Geometry: final body of the model. Coordinates: model frame, mm. A direction names the side the tool comes from. Coordinates: 2 decimals unless noted, no trailing zeros. Order: outer loops, then holes, each group sorted by start corner. A loop starts at its lowest first (then second) coordinate and runs counter-clockwise, first axis right, second up. Notation, with made-up numbers: (59.25, 81.25) -> (100.25, 81.25) arc R8 ccw to (100.25, 88.25) -> close; hole circle Ø6 at (-28, 12.5). An arc over 180 degrees is marked (long way). Answer in a Markdown table with one row per item. Add a question column.
1) Contact query for flat-ended pins moving along their axis: P1, Ø3, axis at x = 4.5, z = 1279, coming from the +Y side; P2, Ø3, axis at x = -44, y = 633.5, coming from the -Z side (3 decimals); P3, Ø6.5, axis at y = 567.5, z = 1304, coming from the +X side. Output: stop coordinate, or through.
2) Pull-direction query (Y, two-part tool) for faces 1 (the face through (41.09, 636, 1326)), 2 (the face through (0.28, 571.68, 1304.63)), 3 (the face through (2.409, 499.464, 1280.401)), 4 (the face through (-42.924, 520.027, 1287.314)); classes: +Y half, -Y half, draft (parallel to the pull), parting line (faces both ways), or undercut.
3) Section query A-A on x = 6.5. Return the cut outline in (y, z), then the cut area to 3 significant figures.
4) Set-up query: faces 5 (the face through (-114.56, 565, 1302)), 6 (the face through (-14.51, 597.37, 1313.26)), 7 (the face through (12.7, 589, 1310)). Return all of +Z, -Z, +X, -X, +Y, -Y with unobstructed straight access to the full face (end or side cutting, diameter ignored); none if empty.
5) Ray query, line 1 (X direction, y = 586, z = 1308); line 2 (Z direction, x = 162.5, y = 593); line 3 (X direction, y = 513.5, z = 1285). Return the intervals inside material, ascending. Write a range as from..to.
```python
from build123d import *

# Parameters (mm, degrees)
SKETCH1_R               = 11.1125
BOSS_EXTRUDE1_DEPTH     = 3.175
F_1_4_20_TAPPED_HOLE1_D = 5.1054
F_10_32_TAPPED_HOLE1_D  = 4.0386
F_8_32_TAPPED_HOLE1_D   = 4.1656
CUT_EXTRUDE1_DEPTH      = 60.342176846
FILLET1_R               = 19.05
F_8_32_TAPPED_HOLE2_D   = 4.1656
F_10_32_TAPPED_HOLE2_D  = 4.1656
SKETCH14_R              = 3.175
SKETCH14_R_2            = 8
SKETCH14_W              = 13
SKETCH14_H              = 20
CUT_EXTRUDE2_DEPTH      = 57.167176846
CUT_EXTRUDE2_DEPTH_BACK = 60.342176846
CUT_EXTRUDE3_START      = -2
CUT_EXTRUDE3_DEPTH      = 2
SKETCH16_R              = 1.5875
CUT_EXTRUDE4_DEPTH      = 58.342176846


with BuildPart() as part:
    # Sketch1 → Boss-Extrude1 (new body)
    with BuildSketch(Plane(origin=(0, -336.500449063, 1001.043483969), x_dir=(-1, 0, 0), z_dir=(0, 0.318629355, -0.947879388))):
        with BuildLine():
            Line((-58.789402849, 930.579137137), (-27.49630657, 876.377904457))
            ThreePointArc((-27.49630657, 876.377904457), (0, 860.502904457), (27.49630657, 876.377904457))
            Line((27.49630657, 876.377904457), (58.789402849, 930.579137137))
            Line((58.789402849, 930.579137137), (185.147535405, 930.579137137))
            Line((185.147535405, 930.579137137), (172.189234839, 989.158155392))
            add(Edge.make_bspline(
                [(172.189234839, 989.158155392), (170.749787142, 995.665292074), (165.52280255, 1008.174916977), (151.405508558, 1023.513956793), (135.711465445, 1031.867037645), (121.896387082, 1035.290959713), (114.765538474, 1035.868385599), (111.210619201, 1035.868385599)],
                knots=[0.20668663, 0.20668663, 0.20668663, 0.20668663, 0.547714054, 0.888741478, 1.229768903, 1.400282615, 1.570796327, 1.570796327, 1.570796327, 1.570796327], degree=3))
            Line((111.210619201, 1035.868385599), (69.85, 1035.868385599))
            Line((69.85, 1035.868385599), (69.85, 1046.47326385))
            Line((69.85, 1046.47326385), (-69.85, 1046.47326385))
            Line((-69.85, 1046.47326385), (-69.85, 1035.868385599))
            Line((-69.85, 1035.868385599), (-111.210619201, 1035.868385599))
            add(Edge.make_bspline(
                [(-172.189234839, 989.158155392), (-170.749787142, 995.665292074), (-165.52280255, 1008.174916977), (-151.405508558, 1023.513956793), (-135.711465445, 1031.867037645), (-121.896387082, 1035.290959713), (-114.765538474, 1035.868385599), (-111.210619201, 1035.868385599)],
                knots=[0.20668663, 0.20668663, 0.20668663, 0.20668663, 0.547714054, 0.888741478, 1.229768903, 1.400282615, 1.570796327, 1.570796327, 1.570796327, 1.570796327], degree=3))
            Line((-172.189234839, 989.158155392), (-185.147535405, 930.579137137))
            Line((-185.147535405, 930.579137137), (-58.789402849, 930.579137137))
        make_face()
        with Locations((0, 892.252904457)):
            Circle(SKETCH1_R, mode=Mode.SUBTRACT)
    extrude(amount=BOSS_EXTRUDE1_DEPTH)

    # 1/4-20 Tapped Hole1 (through all)
    with Locations(Plane(origin=(0, -335.48880086, 998.033966912), x_dir=(-1, 0, 0), z_dir=(0, 0.318629355, -0.947879388))):
        with Locations((82.55, 1029.518385599), (-82.55, 1029.518385599)):
            Hole(F_1_4_20_TAPPED_HOLE1_D / 2)

    # #10-32 Tapped Hole1 (through all)
    with Locations(Plane(origin=(0, -335.48880086, 998.033966912), x_dir=(-1, 0, 0), z_dir=(0, 0.318629355, -0.947879388))):
        with Locations((-18.52177825, 873.731126207), (18.52177825, 873.731126207), (18.52177825, 910.774682707), (-18.52177825, 910.774682707)):
            Hole(F_10_32_TAPPED_HOLE1_D / 2)

    # #8-32 Tapped Hole1 (through all)
    with Locations(Plane(origin=(0, -336.500449063, 1001.043483969), x_dir=(1, 0, 0), z_dir=(0, -0.318629355, 0.947879388))):
        with Locations((63.5, 1040.12326385), (63.5, 951.22326385), (-63.5, 951.22326385), (-63.5, 1040.12326385)):
            Hole(F_8_32_TAPPED_HOLE1_D / 2)

    # Sketch8 → Cut-Extrude1 (cut, through all)
    with BuildSketch(Plane(origin=(0, -335.48880086, 998.033966912), x_dir=(-1, 0, 0), z_dir=(0, 0.318629355, -0.947879388))):
        with BuildLine():
            Line((-41.090457195, 1046.47326385), (-41.090457195, 1004.8172638))
            ThreePointArc((-41.090457195, 1004.8172638), (-35.750879913, 991.926383908), (-22.860000021, 986.586806626))
            Line((-22.860000021, 986.586806626), (-19.05, 986.586806627))
            ThreePointArc((-19.05, 986.586806627), (-14.55987194, 984.726934687), (-12.7, 980.236806627))
            Line((-12.7, 980.236806627), (-12.7, 970.27326385))
            ThreePointArc((-12.7, 970.27326385), (0, 957.57326385), (12.7, 970.27326385))
            Line((12.7, 970.27326385), (12.7, 980.236806629))
            ThreePointArc((12.7, 980.236806629), (14.559871939, 984.726934689), (19.05, 986.586806629))
            Line((19.05, 986.586806629), (22.860000023, 986.586806629))
            ThreePointArc((22.860000023, 986.586806629), (35.75087992, 991.926383918), (41.090457195, 1004.817263822))
            Line((41.090457195, 1004.817263822), (41.0904572, 1046.47326385))
            Line((41.0904572, 1046.47326385), (-41.090457195, 1046.47326385))
        make_face()
    extrude(amount=-CUT_EXTRUDE1_DEPTH, mode=Mode.SUBTRACT)

    # Fillet1
    fillet1_edges = [part.edges().sort_by_distance(p)[0] for p in [
        (-185.147535405, 546.082157979, 1296.048555754),
        (185.147535405, 546.082157979, 1296.048555754),
    ]]
    fillet(fillet1_edges, radius=FILLET1_R)

    # #8-32 Tapped Hole2 (through all)
    with Locations(Plane(origin=(0, -335.48880086, 998.033966912), x_dir=(-1, 0, 0), z_dir=(0, 0.318629355, -0.947879388))):
        with Locations((140.734737002, 936.929137137), (169.906145104, 970.079411683), (150.197707432, 1014.705385734), (107.992809601, 1029.518385599)):
            Hole(F_8_32_TAPPED_HOLE2_D / 2)

    # #10-32 Tapped Hole2 (through all)
    with Locations(Plane(origin=(0, -335.48880086, 998.033966912), x_dir=(-1, 0, 0), z_dir=(0, 0.318629355, -0.947879388))):
        with Locations((-109.05, 975.579137137), (-144.95, 975.579137137)):
            Hole(F_10_32_TAPPED_HOLE2_D / 2)

    # Sketch14 → Cut-Extrude2 (cut, two sides)
    with BuildSketch(Plane(origin=(0, -335.48880086, 998.033966912), x_dir=(-1, 0, 0), z_dir=(0, 0.318629355, -0.947879388))) as cut_extrude2_sk:
        with Locations((123.809674977, 1024.920248146)):
            Circle(SKETCH14_R)
        with Locations((140.734737002, 1017.918189485)):
            Circle(SKETCH14_R)
        with Locations((154.272103769, 1005.5801892)):
            Circle(SKETCH14_R)
        with Locations((162.384030522, 989.158155392)):
            Circle(SKETCH14_R)
        with Locations((161.422942212, 949.629137137)):
            Circle(SKETCH14_R_2)
        with Locations((123.809674977, 949.629137137)):
            Rectangle(SKETCH14_W, SKETCH14_H)
        with BuildLine():
            ThreePointArc((145.026756344, 968.449444325), (140.734737002, 980.539444325), (136.44271766, 968.449444325))
            ThreePointArc((136.44271766, 968.449444325), (140.734737002, 966.925752842), (145.026756344, 968.449444325))
        make_face()
        with BuildLine():
            ThreePointArc((126.779520488, 983.951155392), (123.809674977, 995.152555392), (120.839829466, 983.951155392))
            ThreePointArc((120.839829466, 983.951155392), (123.809674977, 983.163755392), (126.779520488, 983.951155392))
        make_face()
    extrude(amount=CUT_EXTRUDE2_DEPTH, mode=Mode.SUBTRACT)
    extrude(cut_extrude2_sk.sketch, amount=-CUT_EXTRUDE2_DEPTH_BACK, mode=Mode.SUBTRACT)

    # Sketch15 → Cut-Extrude3 (cut)
    with BuildSketch(Plane(origin=(0, -335.48880086, 998.033966912), x_dir=(-1, 0, 0), z_dir=(0, 0.318629355, -0.947879388)).offset(CUT_EXTRUDE3_START)):
        with BuildLine():
            Line((131.059674977, 962.450565709), (116.559674977, 962.450565709))
            ThreePointArc((116.559674977, 962.450565709), (115.145461415, 961.864779271), (114.559674977, 960.450565709))
            Line((114.559674977, 960.450565709), (114.559674977, 939.950565709))
            ThreePointArc((114.559674977, 939.950565709), (115.145461415, 938.536352147), (116.559674977, 937.950565709))
            Line((116.559674977, 937.950565709), (131.059674977, 937.950565709))
            ThreePointArc((131.059674977, 937.950565709), (132.473888539, 938.536352147), (133.059674977, 939.950565709))
            Line((133.059674977, 939.950565709), (133.059674977, 960.450565709))
            ThreePointArc((133.059674977, 960.450565709), (132.473888539, 961.864779271), (131.059674977, 962.450565709))
        make_face()
    extrude(amount=CUT_EXTRUDE3_DEPTH, mode=Mode.SUBTRACT)

    # Sketch16 → Cut-Extrude4 (cut, through all)
    with BuildSketch(Plane(origin=(0, -336.126059571, 999.929725688), x_dir=(-1, 0, 0), z_dir=(0, 0.318629355, -0.947879388))):
        with Locations((118.432206992, 958.506605122)):
            Circle(SKETCH16_R)
        with Locations((129.187142962, 958.506605122)):
            Circle(SKETCH16_R)
        with Locations((129.187142962, 940.751669153)):
            Circle(SKETCH16_R)
        with Locations((118.432206992, 940.751669153)):
            Circle(SKETCH16_R)
    extrude(amount=-CUT_EXTRUDE4_DEPTH, mode=Mode.SUBTRACT)


solid = part.part
```
Result:
| question | item | result |
|---|---|---|
| 1 | P1 | y = 501.37 |
| 1 | P2 | z = 1323.255 |
| 1 | P3 | x = 180.47 |
| 2 | face 1 | draft |
| 2 | face 2 | +Y half |
| 2 | face 3 | undercut |
| 2 | face 4 | -Y half |
| 3 | outline | (479.79, 1275.44) -> (480.8, 1272.43) -> (501.72, 1279.46) -> (500.7, 1282.47) -> close; (517.79, 1288.21) -> (518.8, 1285.2) -> (573.87, 1303.72) -> (572.86, 1306.72) -> close |
| 3 | area | 255 mm2 |
| 4 | face 5 | -Z |
| 4 | face 6 | +Z, +Y |
| 4 | face 7 | +Z, -Z, +Y |
| 5 | line 1 | -175.94..-147.37, -134.1..-12.7, 12.7..175.94 |
| 5 | line 2 | 1310.15..1313.49 |
| 5 | line 3 | -38.93..-10.4, 10.4..38.93 |
